The model under review builds one solid part; all positions refer to its coordinate system, in mm. Face numbers are marked on the shaded views. Give positions to 0.01 mm unless a question says otherwise; leave off trailing zeros. Order: outer loops, then holes, each group sorted by start corner. A loop starts at its lowest first (then second) coordinate and runs counter-clockwise, first axis right, second up. Notation, with made-up numbers: (40, 49.25) - (48, 49.25) arc R19 cw to (48, 71.25) - close; hole circle Ø6 at (-38.5, -34). An arc over 180 degrees is marked (long way). Put each result on its own line as item: value.
```python
from build123d import *

# Parameters (mm, degrees)
F0_R     = 125
F0_R_2   = 120
F1_DEPTH = 250
F3_DEPTH = 8
F4_R     = 174.2845789598
F5_DEPTH = 10


with BuildPart() as f1:
    # F0 (on Top) → F1 (new body)
    with BuildSketch(Plane.XY):
        Circle(F0_R)
        Circle(F0_R_2, mode=Mode.SUBTRACT)
    extrude(amount=F1_DEPTH)

    # F2 (on Top) → F3 (join)
    with BuildSketch(Plane.XY):
        with BuildLine():
            ThreePointArc((14.2534139423, 199.4914539297), (14.8121775768, 201.7984987702), (15, 204.1648029419))
            ThreePointArc((15, 204.1648029419), (-2.3663041716, 218.9769805187), (-14.2534139423, 199.4914539297))
            ThreePointArc((-14.2534139423, 199.4914539297), (0, 200), (14.2534139423, 199.4914539297))
        make_face()
        with BuildLine():
            ThreePointArc((14.2534139423, 199.4914539297), (0, 200), (-14.2534139423, 199.4914539297))
            ThreePointArc((-14.2534139423, 199.4914539297), (0, 189.1648029419), (14.2534139423, 199.4914539297))
        make_face()
        with BuildLine():
            ThreePointArc((14.2534139423, 199.4914539297), (0, 189.1648029419), (-14.2534139423, 199.4914539297))
            ThreePointArc((-14.2534139423, 199.4914539297), (-136.2888792447, -146.3739778589), (200, 0))
            ThreePointArc((200, 0), (146.3739778589, 136.2888792447), (14.2534139423, 199.4914539297))
        make_face()
    extrude(amount=F3_DEPTH)

    # F4 (on face) → F5 (join)
    with BuildSketch(Plane.XY.offset(250)):
        Circle(F4_R)
    extrude(amount=F5_DEPTH)


solid = f1.part
```
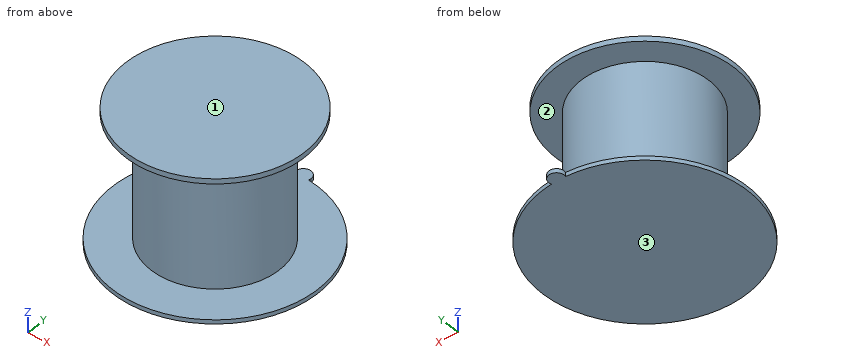
(1) Take a section at C-C, the plane z = 197. Write out the cut boundary in (x, y), then the cut area to 3 significant figures.
The answers:
outline: circle Ø250 at (0, 0); hole circle Ø240 at (0, 0)
area: 3,850 mm^2
(2) Take a section at A-A, the plane y = 0. Write out the cut boundary in (x, z), then the cut area to 3 significant figures.
The answers:
outline: (-200, 0) - (200, 0) - (200, 8) - (125, 8) - (125, 250) - (174.28, 250) - (174.28, 260) - (-174.28, 260) - (-174.28, 250) - (-125, 250) - (-125, 8) - (-200, 8) - close; hole (-120, 8) - (120, 8) - (120, 250) - (-120, 250) - close
area: 9,110 mm^2
(3) Wall thickness on L1, parallel to Z at x = 105, y = 21; L2, parallel to Y at x = 0, z = 158: over which ranges is each line inside the solid? List them lowest first.
The answers:
L1: 0 to 8, 250 to 260
L2: -125 to -120, 120 to 125
(4) Take a section at D-D, the plane y = 187. Write out the cut boundary in (x, z).
The answers:
outline: (-70.93, 0) - (70.93, 0) - (70.93, 8) - (-70.93, 8) - close
(5) Take a section at B-B, the plane x = 0. Write out the cut boundary in (y, z).
The answers:
outline: (-200, 0) - (219.16, 0) - (219.16, 8) - (125, 8) - (125, 250) - (174.28, 250) - (174.28, 260) - (-174.28, 260) - (-174.28, 250) - (-125, 250) - (-125, 8) - (-200, 8) - close; hole (-120, 8) - (120, 8) - (120, 250) - (-120, 250) - close
(6) Clearance check with flat-ended pins moving along their axes: pin 1 Ø3 at (x, z) = (-88.5, 206) entering from +Y; pin 2 Ø12 at (x, z) = (35.5, 64.5) entering from +Y; pin 3 Ø6 at (y, z) = (-65.5, 119) entering from +X. State where each tip first meets the part, or that it passes through.
The answers:
pin 1: y = 89.76
pin 2: y = 121.47
pin 3: x = 108.25
(7) The part is to be moulded in two halves that separate along Z. For the marked faces 1, 2 and 3, say which applies: pulls with the +Z half, pulls with the -Z half, needs draft (parallel to the pull), parting line crosses it, or undercut.
The answers:
face 1: pulls with the +Z half
face 2: undercut
face 3: pulls with the -Z half
